Input: part model. Units: mm. Frame: model coordinates. Face numbers are marked on the shaded views. A direction names the side the tool comes from. Give positions to 0.01 mm unless a question says otherwise; leave off trailing zeros. Order: outer loops, then holes, each group sorted by start corner. A loop starts at its lowest first (then second) coordinate and runs counter-clockwise, first axis right, second up. Notation, with made-up numbers: (76.5, 25.5) - (109.5, 25.5) arc R16 cw to (109.5, 38.5) - close; hole circle Ø4 at (-18.5, 31). An arc over 180 degrees is marked (long way). Use a Markdown table: item, result.
from build123d import *

# Parameters (mm, degrees)
F0_W     = 5
F0_H     = 1
F1_DEPTH = 15
F0_R     = 5.5
F2_DEPTH = 5.5
F3_DEPTH = 2.5


with BuildPart() as f1:
    # F0 (on Top) → F1 (new body)
    with BuildSketch(Plane.XY):
        Rectangle(F0_W, F0_H)
    extrude(amount=F1_DEPTH)

    # F0 (on Top) → F2 (join)
    with BuildSketch(Plane.XY):
        Circle(F0_R)
        Rectangle(F0_W, F0_H, mode=Mode.SUBTRACT)
    extrude(amount=F2_DEPTH)

    # F0 (on Top) → F3 (join)
    with BuildSketch(Plane.XY):
        with BuildLine():
            ThreePointArc((7.7002771781, -0.8764880952), (0, -7.75), (-7.7002771781, -0.8764880952))
            Line((-7.7002771781, -0.8764880952), (-2.980752456, -42.3392857143))
            ThreePointArc((-2.980752456, -42.3392857143), (-0.1699156143, -39.0048157512), (3, -42))
            ThreePointArc((3, -42), (2.9951842488, -42.1699156143), (2.980752456, -42.3392857143))
            Line((2.980752456, -42.3392857143), (7.7002771781, -0.8764880952))
        make_face()
        with BuildLine():
            ThreePointArc((7.7002771781, -0.8764880952), (7.7375593093, -0.4389486702), (7.75, 0))
            ThreePointArc((7.75, 0), (-0.4389486702, 7.7375593093), (-7.7002771781, -0.8764880952))
            ThreePointArc((-7.7002771781, -0.8764880952), (0, -7.75), (7.7002771781, -0.8764880952))
        make_face()
        Circle(F0_R, mode=Mode.SUBTRACT)
        Circle(F0_R)
        Rectangle(F0_W, F0_H, mode=Mode.SUBTRACT)
        with BuildLine():
            ThreePointArc((3, -42), (-0.1699156143, -39.0048157512), (-2.980752456, -42.3392857143))
            ThreePointArc((-2.980752456, -42.3392857143), (0, -45), (2.980752456, -42.3392857143))
            ThreePointArc((2.980752456, -42.3392857143), (2.9951842488, -42.1699156143), (3, -42))
        make_face()
        Rectangle(F0_W, F0_H)
    extrude(amount=-F3_DEPTH)


solid = f1.part
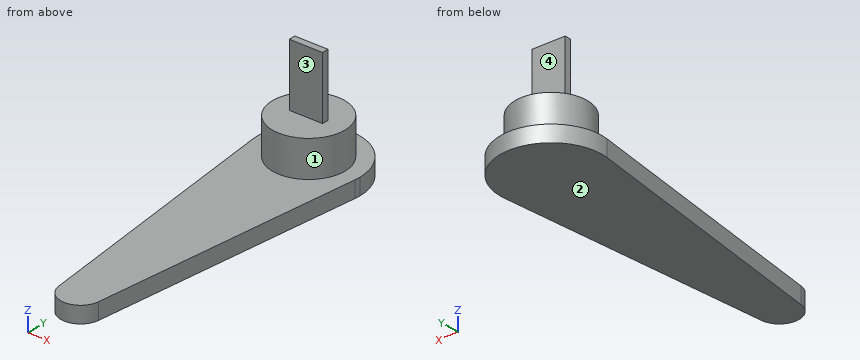
1. Section query B-B (z = 10). Return loops of the section in (x, y).
Response:
| item | result |
|---|---|
| outline | (-2.5, -0.5) - (2.5, -0.5) - (2.5, 0.5) - (-2.5, 0.5) - close |
2. Section query D-D (y = -41). Return loops of the section in (x, z).
Response:
| item | result |
|---|---|
| outline | (-3.13, -2.5) - (3.13, -2.5) - (3.13, 0) - (-3.13, 0) - close |
3. Section query A-A (x = 0). Return loops of the section in (y, z), then the cut area to 3 significant figures.
Response:
| item | result |
|---|---|
| outline | (-45, -2.5) - (7.75, -2.5) - (7.75, 0) - (5.5, 0) - (5.5, 5.5) - (0.5, 5.5) - (0.5, 15) - (-0.5, 15) - (-0.5, 5.5) - (-5.5, 5.5) - (-5.5, 0) - (-45, 0) - close |
| area | 202 mm^2 |
4. Material intervals for line 1 along Y through (x, z) = (-2, 11); line 2 along Z through (x, y) = (-2.5, -11); line 3 along Z through (x, y) = (3.75, -2.5), sorted ascending.
Response:
| item | result |
|---|---|
| line 1 | y = -0.5 to 0.5 |
| line 2 | z = -2.5 to 0 |
| line 3 | z = -2.5 to 5.5 |
5. Pin query (flat end, axial travel): pin 1 (0.5 mm diameter, centred on y = 0, z = 10.5, fed in from +X); pin 2 (4 mm diameter, centred on x = -1, z = 10, fed in from -Y); pin 3 (2.5 mm diameter, centred on x = 0.5, z = 8.5, fed in from +Y); pin 4 (5.5 mm diameter, centred on x = -1, y = -2, fed in from +Z). Return the tip coordinate at first contact, or that it passes through.
Response:
| item | result |
|---|---|
| pin 1 | stops at x = 2.5 |
| pin 2 | stops at y = -0.5 |
| pin 3 | stops at y = 0.5 |
| pin 4 | stops at z = 15 |
6. Section query C-C (x = 3.5). Return loops of the section in (y, z), then the cut area to 3 significant figures.
Response:
| item | result |
|---|---|
| outline | (-37.78, -2.5) - (6.91, -2.5) - (6.91, 0) - (4.24, 0) - (4.24, 5.5) - (-4.24, 5.5) - (-4.24, 0) - (-37.78, 0) - close |
| area | 158 mm^2 |
7. Set-up query: the marked faces 1, 2, 3 and 4. Return all of +Z, -Z, +X, -X, +Y, -Y with unobstructed straight access to the full face (end or side cutting, diameter ignored); none if empty.
Response:
| item | result |
|---|---|
| face 1 | +Z |
| face 2 | -Z, +X, -X, +Y, -Y |
| face 3 | +Z, +X, -X, -Y |
| face 4 | +Z, +X, -X, +Y |
